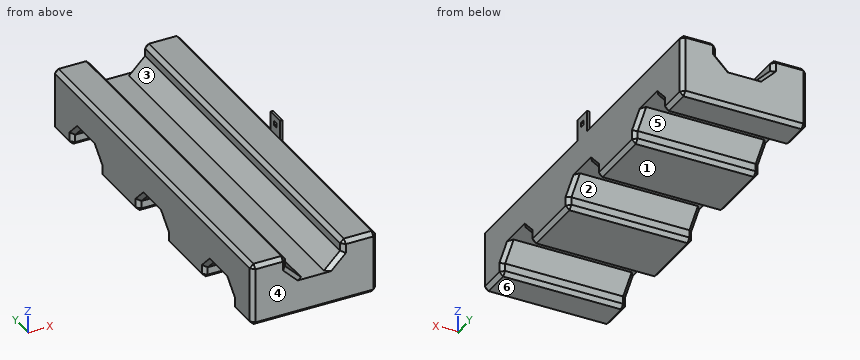
from build123d import *

# Parameters (mm, degrees)
SKETCH1_W                = 50
SKETCH1_H                = 150
BOSS_EXTRUDE1_DEPTH      = 25
CUT_EXTRUDE1_DEPTH       = 161.078105936
CUT_EXTRUDE2_DEPTH       = 161.078105936
LPATTERN1_COUNT          = 3
LPATTERN1_PITCH          = 50
CHAMFER1_SIZE            = 1.5
BOSS_EXTRUDE2_DEPTH      = 7
BOSS_EXTRUDE2_DEPTH_BACK = 10
SKETCH4_W                = 1
SKETCH4_H                = 7
SKETCH5_W                = 1.8
SKETCH5_H                = 1.8
CUT_EXTRUDE3_DEPTH       = 7


with BuildPart() as part:
    # Sketch1 → Boss-Extrude1 (new body)
    with BuildSketch(Plane.XY):
        with Locations((25, 75)):
            Rectangle(SKETCH1_W, SKETCH1_H)
    extrude(amount=BOSS_EXTRUDE1_DEPTH)

    # Sketch2 → Cut-Extrude1 (cut, through all)
    with BuildSketch(Plane.XZ):
        Polygon((29.556349186, 36), (20.443650814, 36), (14, 29.556349186), (14, 20.443650814), (20.443650814, 14), (29.556349186, 14), (36, 20.443650814), (36, 29.556349186), align=None)
    extrude(amount=-CUT_EXTRUDE1_DEPTH, mode=Mode.SUBTRACT)

    # Sketch3 → Cut-Extrude2 (cut, through all)
    with BuildSketch(Plane(origin=(50, 0, 0), x_dir=(0, 0, -1), z_dir=(1, 0, 0))):
        Polygon((-4.556349186, 36), (-11, 29.556349186), (-11, 20.443650814), (-4.556349186, 14), (4.556349186, 14), (11, 20.443650814), (11, 29.556349186), (4.556349186, 36), align=None)
    cut_extrude2 = extrude(amount=-CUT_EXTRUDE2_DEPTH, mode=Mode.SUBTRACT)

    # LPattern1: Cut-Extrude2 ×3
    with Locations(*[(0, i * LPATTERN1_PITCH, 0) for i in range(1, LPATTERN1_COUNT)]):
        add(cut_extrude2, mode=Mode.SUBTRACT)

    # Chamfer1
    chamfer1_edges = [part.edges().sort_by_distance(p)[0] for p in [
        (50, 75, 25),
        (50, 143, 0),
        (50, 136, 2.278174593),
        (0, 100, 0),
        (25, 136, 0),
        (25, 114, 0),
        (0, 136, 2.278174593),
        (0, 114, 2.278174593),
        (0, 117.221825407, 7.778174593),
        (0, 132.778174593, 7.778174593),
        (50, 132.778174593, 7.778174593),
        (50, 117.221825407, 7.778174593),
        (50, 114, 2.278174593),
        (43, 150, 25),
        (43, 0, 25),
        (7, 150, 25),
        (14, 75, 25),
        (36, 75, 25),
        (36, 150, 22.721825407),
        (14, 150, 22.721825407),
        (36, 0, 22.721825407),
        (14, 0, 22.721825407),
        (17.221825407, 0, 17.221825407),
        (32.778174593, 0, 17.221825407),
        (32.778174593, 150, 17.221825407),
        (17.221825407, 150, 17.221825407),
        (0, 75, 25),
        (25, 150, 0),
        (50, 7, 0),
        (25, 0, 0),
        (0, 7, 0),
        (50, 50, 0),
        (25, 14, 0),
        (25, 36, 0),
        (0, 143, 0),
        (0, 36, 2.278174593),
        (0, 14, 2.278174593),
        (0, 17.221825407, 7.778174593),
        (0, 32.778174593, 7.778174593),
        (50, 36, 2.278174593),
        (50, 32.778174593, 7.778174593),
        (50, 17.221825407, 7.778174593),
        (50, 14, 2.278174593),
        (7, 0, 25),
        (0, 150, 12.5),
        (50, 150, 12.5),
        (50, 0, 12.5),
        (0, 0, 12.5),
        (50, 100, 0),
        (50, 86, 2.278174593),
        (0, 50, 0),
        (25, 86, 0),
        (25, 64, 0),
        (0, 86, 2.278174593),
        (0, 64, 2.278174593),
        (0, 67.221825407, 7.778174593),
        (0, 82.778174593, 7.778174593),
        (50, 82.778174593, 7.778174593),
        (50, 67.221825407, 7.778174593),
        (50, 64, 2.278174593),
    ]]
    chamfer(chamfer1_edges, length=CHAMFER1_SIZE)

    # Sketch4 → Boss-Extrude2 (add, two sides: drawn at the far end of the back side and taken through both)
    with BuildSketch(Plane.XY.offset(25).offset(-BOSS_EXTRUDE2_DEPTH_BACK)):
        with Locations((49.5, 75)):
            Rectangle(SKETCH4_W, SKETCH4_H)
    extrude(amount=BOSS_EXTRUDE2_DEPTH + BOSS_EXTRUDE2_DEPTH_BACK)

    # Sketch5 → Cut-Extrude3 (cut)
    with BuildSketch(Plane(origin=(50, 0, 0), x_dir=(0, 0, -1), z_dir=(1, 0, 0))):
        with Locations((-28.6, 75)):
            Rectangle(SKETCH5_W, SKETCH5_H)
    extrude(amount=-CUT_EXTRUDE3_DEPTH, mode=Mode.SUBTRACT)


solid = part.part
Model file for the job. Use its own axes, mm. Face numbers are marked on the shaded views. A direction names the side the tool comes from. Give positions to 0.01 mm unless a question says otherwise; leave off trailing zeros. Order: outer loops, then holes, each group sorted by start corner. A loop starts at its lowest first (then second) coordinate and runs counter-clockwise, first axis right, second up. Notation, with made-up numbers: (24, 87.5) -> (53, 87.5) arc R5 cw to (53, 92.5) -> close; hole circle Ø6 at (53.5, 8). An arc over 180 degrees is marked (long way). Use CSV: the item, a comma, the result in double quotes.
1. Drop flat-ended pins along their axis: pin 1 (1.1 mm diameter, centred on x = 49.5, y = 75, fed in from -Z); pin 2 (14.5 mm diameter, centred on x = 25.5, y = 28, fed in from -Z); pin 3 (12 mm diameter, centred on x = 35, y = 20.5, fed in from -Z); pin 4 (1 mm diameter, centred on x = 16, z = 24.5, fed in from -Y). Give the stop position or say it passes through.
Outcome:
pin 1,"z = 11"
pin 2,"z = 5.31"
pin 3,"z = 5.06"
pin 4,"through"
2. Band-saw the part on C-C, the plane y = 96. Give the cut face in (x, z), then the cut area to 3 significant figures.
Outcome:
outline,"(0, 1.5) -> (1.5, 0) -> (48.5, 0) -> (50, 1.5) -> (50, 23.5) -> (48.5, 25) -> (37.5, 25) -> (36, 23.5) -> (36, 20.44) -> (29.56, 14) -> (20.44, 14) -> (14, 20.44) -> (14, 23.5) -> (12.5, 25) -> (1.5, 25) -> (0, 23.5) -> close"
area,"1,040 mm²"
3. Band-saw the part on A-A, the plane z = 22. Give the cut face in (x, y).
Outcome:
outline,"(0, 1.5) -> (1.5, 0) -> (12.5, 0) -> (14, 1.5) -> (14, 148.5) -> (12.5, 150) -> (1.5, 150) -> (0, 148.5) -> close; (36, 1.5) -> (37.5, 0) -> (48.5, 0) -> (50, 1.5) -> (50, 148.5) -> (48.5, 150) -> (37.5, 150) -> (36, 148.5) -> close"
4. Band-saw the part on D-D, the plane z = 7.5. Count the separate pieces of the cut face and the enclosed holes in it, then the cut area to 3 significant figures.
Outcome:
separate pieces,"4"
enclosed holes,"0"
area,"5,060 mm²"
5. Drill centre lines: line 1 along Y through (x, z) = (34, 3); line 2 along Y through (x, z) = (3, 5); line 3 along X through (y, z) = (102.5, 22). Where is each one in solid material? Low to high. Write a range as from..to.
Outcome:
line 1,"0..14, 36..64, 86..114, 136..150"
line 2,"0..14.44, 35.56..64.44, 85.56..114.44, 135.56..150"
line 3,"0..14, 36..50"
6. Mould opens along Y. For the marked faces 4, 5 and 6 say: +Y half, -Y half, draft (parallel to the pull), parting line (faces both ways), or undercut.
Outcome:
face 4,"-Y half"
face 5,"undercut"
face 6,"draft"
7. 3-axis set-ups, long thin cutter, end or side, ignore diameter. For the marked faces 1, 2 and 3: which of +Z, -Z, +X, -X, +Y, -Y reach the whole face in a straight line?
Outcome:
face 1,"-Z, +X, -X, +Y, -Y"
face 2,"-Z, +X, -X"
face 3,"+Z, +Y, -Y"
